Source: CAD feature listing. Evaluate the final solid. Frame: model axes, mm. Face numbers are marked on the shaded views. A direction names the side the tool comes from. Coordinates: 2 decimals unless noted, no trailing zeros. Order: outer loops, then holes, each group sorted by start corner. A loop starts at its lowest first (then second) coordinate and runs counter-clockwise, first axis right, second up. Notation, with made-up numbers: (67.5, 78) - (105.5, 78) arc R20 cw to (105.5, 95) - close; hole circle Ø6 at (71, 81). An arc over 180 degrees is marked (long way). One line per question, with ' | ' between items. Start each with the question number.
(1) Section A-A (x = -50). Return the cut outline in (y, z), then the cut area to 3 significant figures.
(2) Contact query for flat-ended pins moving along their axis: P1, Ø8, axis at x = 0, z = 0, coming from the +Y side; P2, Ø22.5, axis at y = 101, z = -12, coming from the -X side. Output: stop coordinate, or through.
(3) Section D-D (x = 9.5). Return the cut outline in (y, z).
(4) Section C-C (y = 87.5). Return the cut outline in (x, z).
(5) Access query for the marked faces 1 and 2. Directions: +Z, -Z, +X, -X, +Y, -Y. A direction counts if a zero-diameter tool reaches every point of the face in a straight line with its end or side. Return the directions, or none.
(6) Section B-B (z = -21). Return the cut outline in (x, y).
(7) Line query: line 1 along X through (y, z) = (6, 0); line 2 along X through (y, z) = (123.5, 5.5); line 3 along Y through (x, z) = (-48, 17). Output: solid intervals per line, ascending.
from build123d import *

# Parameters (mm, degrees)
ANGULO_L_DEPTH             = 37.5
CROQUIS_AGUJEROS_MONTAJE_R = 5
AGUJERO_INSERTO_M6_DEPTH   = 14


with BuildPart() as part:
    # Croquis_perfil_L → Angulo_L (new, symmetric)
    with BuildSketch(Plane.XY):
        Polygon((-62.5, 0), (62.5, 0), (62.5, 150), (37.5, 150), (37.5, 20), (-62.5, 20), align=None)
    extrude(amount=ANGULO_L_DEPTH, both=True)

    # Croquis_agujeros_montaje → Agujero_inserto_M6 (cut)
    with BuildSketch(Plane(origin=(0, 0, 0), x_dir=(1, 0, 0), z_dir=(0, 1, 0))):
        with Locations(Location((-50, 0, 0), (0, 0, 270))):
            Circle(CROQUIS_AGUJEROS_MONTAJE_R)
        with Locations(Location((0, 0, 0), (0, 0, 270))):
            Circle(CROQUIS_AGUJEROS_MONTAJE_R)
    extrude(amount=AGUJERO_INSERTO_M6_DEPTH, mode=Mode.SUBTRACT)


solid = part.part
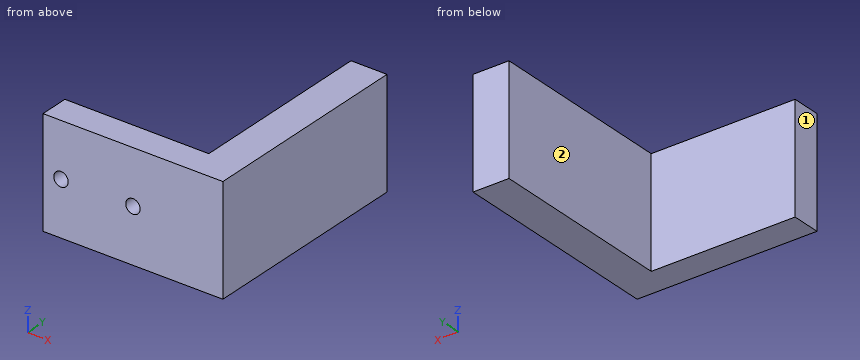
Response values:
1) outline: (0, -37.5) - (20, -37.5) - (20, 37.5) - (0, 37.5) - (0, 5) - (14, 5) - (14, -5) - (0, -5) - close | area: 1,360 mm²
2) P1: stops at y = 20 | P2: stops at x = 37.5
3) outline: (0, -37.5) - (20, -37.5) - (20, 37.5) - (0, 37.5) - close
4) outline: (37.5, -37.5) - (62.5, -37.5) - (62.5, 37.5) - (37.5, 37.5) - close
5) face 1: +Z, -Z, -X, +Y, -Y | face 2: +Z, -Z, -X, +Y
6) outline: (-62.5, 0) - (62.5, 0) - (62.5, 150) - (37.5, 150) - (37.5, 20) - (-62.5, 20) - close
7) line 1: x = -62.5 to -55, -45 to -5, 5 to 62.5 | line 2: x = 37.5 to 62.5 | line 3: y = 0 to 20
